Geometry check sheet. Reference: the model listing, model coordinates, mm. Face numbers are marked on the shaded views. A direction names the side the tool comes from. Give positions to 0.01 mm unless a question says otherwise; leave off trailing zeros. Order: outer loops, then holes, each group sorted by start corner. A loop starts at its lowest first (then second) coordinate and runs counter-clockwise, first axis right, second up. Notation, with made-up numbers: M 56.25,15.25 L 105.25,15.25 A22 cw 105.25,43.25 Z; hole C 24.25,11 d2. An arc over 180 degrees is marked long. Answer as a JSON object with one key per item and string values. Group by question number.
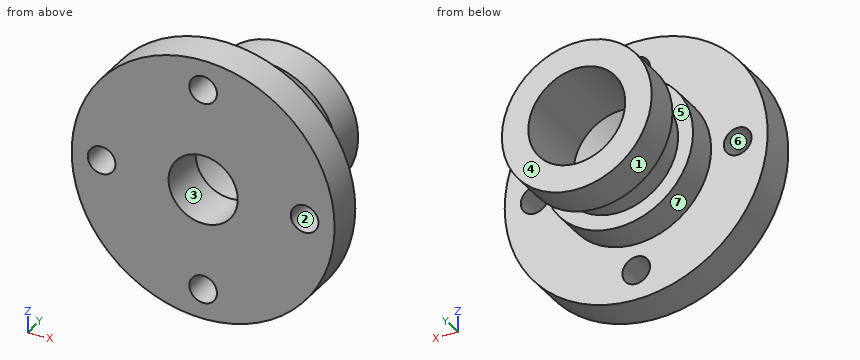
from build123d import *

# Parameters (mm, degrees)
SKETCH_6_R               = 6
CUT_EXTRUDE_2_DEPTH      = 63
PATTERN_CIRCULAR_1_COUNT = 4


with BuildPart() as part:
    # 스케치2 → 회전1 (revolve)
    with BuildSketch(Plane.XY):
        Polygon((0, 0), (57, 0), (57, 16), (32.5, 16), (32.5, 30), (26, 30), (26, 46), (32.5, 46), (32.5, 62), (0, 62), align=None)
    revolve(axis=Axis((0, 81.32, 0), (0, -1, 0)))

    # 스케치5 → 컷-회전1 (revolve, cut)
    with BuildSketch(Plane.XY):
        Polygon((0, 0), (15, 0), (15, 21), (21, 27), (21, 62), (0, 62), align=None)
    revolve(axis=Axis((0, 62, 0), (0, -1, 0)), mode=Mode.SUBTRACT)

    # 스케치6 → 컷-돌출2 (cut, through all)
    with BuildSketch(Plane(origin=(0, 0, 0), x_dir=(1, 0, 0), z_dir=(0, 1, 0))):
        with Locations((0, 44)):
            Circle(SKETCH_6_R)
    cut_extrude_2 = extrude(amount=CUT_EXTRUDE_2_DEPTH, mode=Mode.SUBTRACT)

    # 원형 패턴1: 컷-돌출2 ×4 about axis
    pattern_circular_1_axis = Axis((0, 0, 0), (0, 1, 0))
    for i in range(1, PATTERN_CIRCULAR_1_COUNT):
        add(cut_extrude_2.rotate(pattern_circular_1_axis, i * 360 / PATTERN_CIRCULAR_1_COUNT), mode=Mode.SUBTRACT)


solid = part.part
1. Cross-section at B-B (y = 9.5). Record the cut outline in (x, z), and give its area (3 significant figures).
2. Access from +Z, -Z, +X, -X, +Y, -Y to the whole of each face (thin tool, end or side, straight path). Record for the marked faces 5, 6 and 7.
3. Cross-section at D-D (x = -44). Record the cut outline in (y, z), and give its area (3 significant figures).
4. Thickness scan on line 1 along Y through (x, z) = (31, 8); line 2 along Z through (x, y) = (5, 15); line 3 along Z through (x, y) = (-12.5, 20). Record the ranges inside material, lowest first. Write a range as [from, to].
5. Cross-section at A-A (z = 0). State how many separate pieces and enclosed holes the cut face has, and give its area (3 significant figures).
6. Depth check by flat-ended pin: pin 1 (3 mm diameter, centred on y = 20.5, z = 19.5, fed in from -X); pin 2 (1 mm diameter, centred on x = -44.5, y = 15.5, fed in from +Z); pin 3 (8 mm diameter, centred on x = 3.5, y = 46, fed in from +Z). Enter the tip coordinate at first touch or a pass-through.
7. Cross-section at C-C (z = -44). Record the cut outline in (x, y).
8. Release check for a two-part mould opening along Z. For the marked faces 1, 2, 3 and 4 record: released by +Z, released by -Z, zero draft, split by the parting line, or undercut.
Report:
{
 "1": {"outline": "C 0,0 d114; hole C -44,0 d12; hole C 0,0 d30; hole C 0,-44 d12; hole C 0,44 d12; hole C 44,0 d12", "area": "9,050 mm2"},
 "2": {"face 5": "none", "face 6": "+Y, -Y", "face 7": "+Y"},
 "3": {"outline": "M 0,-36.24 L 16,-36.24 L 16,-6 L 0,-6 Z; M 0,6 L 16,6 L 16,36.24 L 0,36.24 Z", "area": "968 mm2"},
 "4": {"line 1": "y = [0, 30], [46, 62]", "line 2": "z = [-56.78, -47.32], [-40.68, -14.14], [14.14, 40.68], [47.32, 56.78]", "line 3": "z = [-30, -8.29], [8.29, 30]"},
 "5": {"separate pieces": "4", "enclosed holes": "0", "area": "1,910 mm2"},
 "6": {"pin 1": "stops at x = -27.06", "pin 2": "stops at z = 36.24", "pin 3": "stops at z = 32.5"},
 "7": {"outline": "M -36.24,0 L -6,0 L -6,16 L -36.24,16 Z; M 6,0 L 36.24,0 L 36.24,16 L 6,16 Z"},
 "8": {"face 1": "split by the parting line", "face 2": "undercut", "face 3": "undercut", "face 4": "zero draft"}
}
